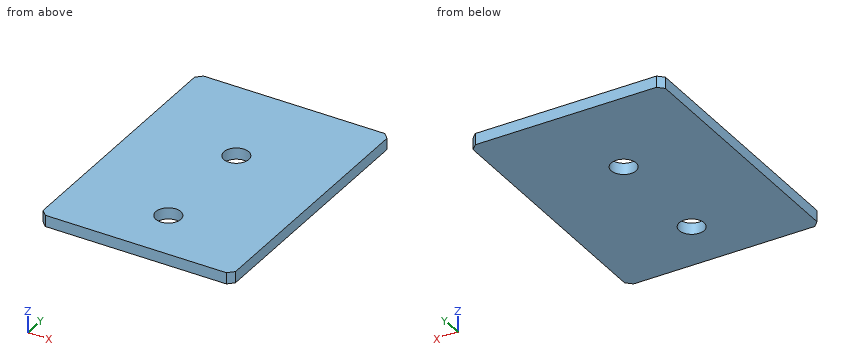
```python
from build123d import *

# Parameters (mm, degrees)
SKETCH1_W           = 170
SKETCH1_H           = 232.717889213
SKETCH1_R           = 11
BOSS_EXTRUDE1_DEPTH = 10
CHAMFER1_SIZE       = 5


with BuildPart() as part:
    # Sketch1 → Boss-Extrude1 (new body)
    with BuildSketch(Plane.XY):
        with Locations((0, -31.358944607)):
            Rectangle(SKETCH1_W, SKETCH1_H)
        Circle(SKETCH1_R, mode=Mode.SUBTRACT)
        with Locations((0, -100)):
            Circle(SKETCH1_R, mode=Mode.SUBTRACT)
    extrude(amount=BOSS_EXTRUDE1_DEPTH)

    # Chamfer1
    chamfer1_edges = [part.edges().sort_by_distance(p)[0] for p in [
        (-85, 85, 5),
        (85, 85, 5),
        (85, -147.717889213, 5),
        (-85, -147.717889213, 5),
    ]]
    chamfer(chamfer1_edges, length=CHAMFER1_SIZE)


solid = part.part
```
Geometry check sheet. Reference: the model listing, model coordinates, mm. Coordinates: 2 decimals unless noted, no trailing zeros. Write each loop counter-clockwise with the first axis right and the second up, starting at its lowest first coordinate (ties: lowest second). Pieces come first, ordered by that corner, then holes. Notation, with made-up numbers: M 22.25,-17 L 45.25,-17 A25 cw 45.25,1 Z; hole C 49,86 d9. An arc over 180 degrees is marked long. Answer as a JSON object with one key per item and string values.
1. Section check B-B, the plane x = 0. Enter the section's corners in (y, z).
Answers below:
{"outline": "M -147.72,0 L -111,0 L -111,10 L -147.72,10 Z; M -89,0 L -11,0 L -11,10 L -89,10 Z; M 11,0 L 85,0 L 85,10 L 11,10 Z"}
2. Scan lines: L1, parallel to Y at x = 0, z = 2.75; L2, parallel to X at y = -100.5, z = 0.5; L3, parallel to X at y = 8.5, z = 6. Record each from-to range of solid material in increasing order.
Answers below:
{"L1": "y = -147.72 to -111, -89 to -11, 11 to 85", "L2": "x = -85 to -10.99, 10.99 to 85", "L3": "x = -85 to -6.98, 6.98 to 85"}
3. Section check C-C, the plane z = 7. Enter the section's corners in (x, y).
Answers below:
{"outline": "M -85,-142.72 L -80,-147.72 L 80,-147.72 L 85,-142.72 L 85,80 L 80,85 L -80,85 L -85,80 Z; hole C 0,-100 d22; hole C 0,0 d22"}
4. Section check D-D, the plane y = 6. Enter the section's corners in (x, z), plus the area to 3 significant figures.
Answers below:
{"outline": "M -85,0 L -9.22,0 L -9.22,10 L -85,10 Z; M 9.22,0 L 85,0 L 85,10 L 9.22,10 Z", "area": "1,520 mm²"}
5. Section check A-A, the plane y = -100. Enter the section's corners in (x, z), plus the area to 3 significant figures.
Answers below:
{"outline": "M -85,0 L -11,0 L -11,10 L -85,10 Z; M 11,0 L 85,0 L 85,10 L 11,10 Z", "area": "1,480 mm²"}
6. Go/stop test with a flat-tipped pin: pin 1 Ø10 at (x, y) = (-10, -46) entering from -Z. Record where the tip stops, or that it passes through.
Answers below:
{"pin 1": "stops at z = 0"}
